Autodesk Inventor part; units mm, degrees
ref_plane "YZ Plane" through (0, 0, 0) normal (1, 0, 0) x (0, 1, 0)
ref_plane "XZ Plane" through (0, 0, 0) normal (0, 1, 0) x (-1, 0, 0)
ref_plane "XY Plane" through (0, 0, 0) normal (0, 0, 1) x (1, 0, 0)
sketch "스케치1" plane through (0, 0, 0) normal (0, 0, 1) x (1, 0, 0)
  line L0 (0, 0) -> (40, 0)
  line L1 (40, 0) -> (40, 36.6)
  line L2 (40, 36.6) -> (0, 36.6)
  line L3 (0, 36.6) -> (0, 0)
  dimension "d0" = 40
  dimension "d1" = 36.6
extrude "돌출1" add sketch "스케치1" along normal blind 20
sketch "스케치2" plane through (0, 0, 20) normal (0, 0, 1) x (1, 0, 0)
  line L0 (40, 0) -> (40, 36.6)
  line L1 (40, 30.5) -> (46.85, 30.5)
  line L2 (46.85, 30.5) -> (46.85, 28.2)
  line L3 (46.85, 28.2) -> (40, 28.2)
  line L4 (40, 28.2) -> (40, 30.5)
  line L5 (0, 30.5) -> (-6.85, 30.5)
  line L6 (-6.85, 30.5) -> (-6.85, 28.2)
  line L7 (-6.85, 28.2) -> (0, 28.2)
  line L8 (0, 28.2) -> (0, 30.5)
  line L9 (0, 0) -> (40, 0)
  line L10 (0, 36.6) -> (0, 0)
  point P0 (40, 28.2)
  point P1 (0, 29.35)
  dimension "d4" = 6.85
  dimension "d5" = 6.85
  dimension "d6" = 2.3
  dimension "d7" = 2.3
  dimension "d8" = 30.5
  dimension "d9" = 30.5
extrude "돌출2" add sketch "스케치2" against normal blind 20
sketch "스케치3" plane through (0, 36.6, 0) normal (0, 1, 0) x (1, 0, 0)
  line L0 (40, 0) -> (0, 0)
  line L1 (0, 0) -> (0, -20)
  line L2 (40, -20) -> (0, -20)
  line L3 (40, 0) -> (40, -20)
  circle A0 centre (10, -10) radius 10
  line L4 (0, 0) -> (0, -20)
  line L5 (0, -20) -> (34.3, -20)
  line L6 (34.3, -20) -> (34.3, 0)
  line L7 (34.3, 0) -> (0, 0)
  line L8 (0, 0) -> (0, -20)
  line L9 (40, -20) -> (0, -20)
  point P0 (10, -20)
  point P1 (10, 0)
  dimension "d12" = 34.3
extrude "돌출3" add sketch "스케치3" along normal blind 2.7 contours L6 L2 A0 L0 | A0
sketch "스케치4" plane through (0, 39.3, 0) normal (0, 1, 0) x (1, 0, 0)
  circle A0 centre (9.15, -10) radius 2.5
  arc A1 (10, 0) -> (10, -20) centre (10, -10) ccw
  line L0 (-6.85, -20) -> (-6.85, 0)
  point P0 (0, 0)
  point P1 (0, -10)
  point P2 (11.638, -9.755)
  point P3 (0, -10)
  point P4 (0, -10)
  dimension "d15" = 5
  dimension "d23" = 16
extrude "돌출4" add sketch "스케치4" along normal blind 5.5
sketch "스케치5" plane through (0, 39.3, 0) normal (0, 1, 0) x (1, 0, 0)
  circle A0 centre (9.15, -10) radius 2.5
  line L0 (10, -20) -> (34.3, -20)
  line L1 (34.3, -20) -> (34.3, 0)
  line L2 (34.3, 0) -> (10, 0)
  arc A1 (10, 0) -> (10, -20) centre (10, -10) ccw
  circle A2 centre (10, -10) radius 7.5
  point P0 (0, 0)
  dimension "d20" = 15
sketch "스케치6" plane through (0, 0, 20) normal (0, 0, 1) x (1, 0, 0)
  point P0 (0, 0)
extrude "돌출5" add sketch "스케치5" along normal blind 1.3 contours A2
sketch "스케치18" plane through (0, 39.3, 0) normal (0, 1, 0) x (1, 0, 0)
  point P0 (0, 0)
sketch "스케치19" plane through (40, 30.5, 20) normal (0, 1, 0) x (1, 0, 0)
  circle A0 centre (4.5, 15) radius 2
  circle A1 centre (4.5, 5) radius 2
  line L0 (6.85, 0) -> (0, 0)
  line L1 (6.85, 0) -> (6.85, 20)
  line L2 (0, 20) -> (6.85, 20)
  line L3 (0, 0) -> (0, 20)
  circle A2 centre (-30, 10) radius 7.5
  line L4 (-30, 0) -> (-5.7, 0)
  line L5 (-5.7, 0) -> (-5.7, 20)
  line L6 (-5.7, 20) -> (-30, 20)
  arc A3 (-30, 20) -> (-30, 0) centre (-30, 10) ccw
  line L7 (-17.85, 0) -> (-17.85, 20)
  circle A4 centre (-44.5, 15) radius 2
  line L8 (-46.85, 0) -> (-46.85, 20)
  circle A5 centre (-44.5, 5) radius 2
  line L9 (-46.85, 20) -> (-40, 20)
  dimension "d24" = 4
  dimension "d25" = 4
  dimension "d26" = 10
  dimension "d27" = 5
  dimension "d29" = 2.35
  dimension "d30" = 4
  dimension "d31" = 2.35
  dimension "d32" = 2.35
  dimension "d33" = 4
  dimension "d34" = 2.35
  dimension "d35" = 10
  dimension "d36" = 5
extrude "돌출6" cut sketch "스케치19" against normal through all contours A0 | A1 | A4 | A5
sketch "스케치35" plane through (0, 0, 0) normal (0, -1, 0) x (1, 0, 0)
  circle A0 centre (9.15, 10) radius 2.5
  circle A1 centre (9.15, 10) radius 10.5
  point P0 (0, 0)
  dimension "d39" = 21
sketch "스케치36" plane through (0, 0, 20) normal (0, 0, 1) x (1, 0, 0)
  line L0 (40, 0) -> (40, 28.2)
  line L1 (40, 28.2) -> (46.85, 28.2)
  line L2 (46.85, 28.2) -> (46.85, 30.5)
  line L3 (46.85, 30.5) -> (40, 30.5)
  line L4 (40, 30.5) -> (40, 36.6)
  line L5 (40, 36.6) -> (34.3, 36.6)
  line L6 (34.3, 36.6) -> (34.3, 39.3)
  line L7 (10, 39.3) -> (34.3, 39.3)
  line L8 (10, 36.6) -> (10, 39.3)
  line L9 (10, 36.6) -> (0, 36.6)
  line L10 (0, 36.6) -> (0, 30.5)
  line L11 (0, 30.5) -> (-6.85, 30.5)
  line L12 (-6.85, 30.5) -> (-6.85, 28.2)
  line L13 (-6.85, 28.2) -> (0, 28.2)
  line L14 (0, 28.2) -> (0, 0)
  line L15 (0, 0) -> (40, 0)
properties part number "996R모터_3D 인쇄"
CAD build for the part. Positions are in the model's coordinates, mm. A direction names the side the tool comes from. Coordinates: 2 decimals unless noted, no trailing zeros. Order: outer loops, then holes, each group sorted by start corner. A loop starts at its lowest first (then second) coordinate and runs counter-clockwise, first axis right, second up. Notation, with made-up numbers: M 18.25,-7.5 L 68.25,-7.5 A17 cw 68.25,-2.5 Z; hole C 66,68.25 d5. An arc over 180 degrees is marked long. Answer as CSV lines item,"result".
1) Flat gauge pins, fed straight in: P1, Ø8, axis at x = 7, z = 17, coming from the +Y side; P2, Ø5, axis at x = 35.5, z = 9, coming from the +Y side; P3, Ø4.5, axis at x = 44.5, z = 5, coming from the +Y side. Where does each tip first touch, or does it go through?
Verdict:
P1,"y = 40.6"
P2,"y = 39.3"
P3,"y = 30.5"
2) Drill centre lines: L1, parallel to Z at x = 44.5, y = 29.05; L2, parallel to X at y = 28.8, z = 15; L3, parallel to Y at x = 15, z = 11.75. Where is each one in solid material? Low to high. Write a range as from..to.
Verdict:
L1,"0..3, 7..13, 17..20"
L2,"-6.85..-6.5, -2.5..42.5, 46.5..46.85"
L3,"0..40.6"
3) Mould opens along Z. For faces 5 (the flat face through (21, 39.3, 10)), 6 (the flat face through (20, 20, 20)), 7 (the cylindrical face through (-4.76, 29.366, 13.017)) say: released by +Z, released by -Z, zero draft, split by the parting line, or undercut.
Verdict:
face 5,"zero draft"
face 6,"released by +Z"
face 7,"undercut"
4) 3-axis set-ups, long thin cutter, end or side, ignore diameter. For faces 1 (the flat face through (2, 36.6, 18)), 2 (the flat face through (-3, 28.2, 10)), 3 (the flat face through (2, 36.6, 2)), 4 (the cylindrical face through (8.61, 42.67, 7.56)): which of +Z, -Z, +X, -X, +Y, -Y reach the whole face in a straight line?
Verdict:
face 1,"+Z, -X, +Y"
face 2,"+Z, -Z, -X, -Y"
face 3,"-Z, -X, +Y"
face 4,"+Y"
5) Cut at C-C (x = 14). List the corners of the cut face in (y, z), then the cut area to 3 significant figures.
Verdict:
outline,"M 0,0 L 39.3,0 L 39.3,3.66 L 40.6,3.66 L 40.6,16.34 L 39.3,16.34 L 39.3,20 L 0,20 Z"
area,"802 mm2"
6) Cut at A-A (x = 44.5). List the corners of the cut face in (y, z).
Verdict:
outline,"M 28.2,0 L 30.5,0 L 30.5,3 L 28.2,3 Z; M 28.2,7 L 30.5,7 L 30.5,13 L 28.2,13 Z; M 28.2,17 L 30.5,17 L 30.5,20 L 28.2,20 Z"
7) Cut at B-B (z = 15). List the corners of the cut face in (x, y).
Verdict:
outline,"M -6.85,28.2 L -6.5,28.2 L -6.5,30.5 L -6.85,30.5 Z; M -2.5,28.2 L 0,28.2 L 0,0 L 40,0 L 40,28.2 L 42.5,28.2 L 42.5,30.5 L 40,30.5 L 40,36.6 L 34.3,36.6 L 34.3,39.3 L 15.59,39.3 L 15.59,40.6 L 4.41,40.6 L 4.41,39.3 L 1.34,39.3 L 1.34,36.6 L 0,36.6 L 0,30.5 L -2.5,30.5 Z; M 46.5,28.2 L 46.85,28.2 L 46.85,30.5 L 46.5,30.5 Z"
8) Cut at D-D (y = 4.5). List the corners of the cut face in (x, z), then the cut area to 3 significant figures.
Verdict:
outline,"M 0,0 L 40,0 L 40,20 L 0,20 Z"
area,"800 mm2"
